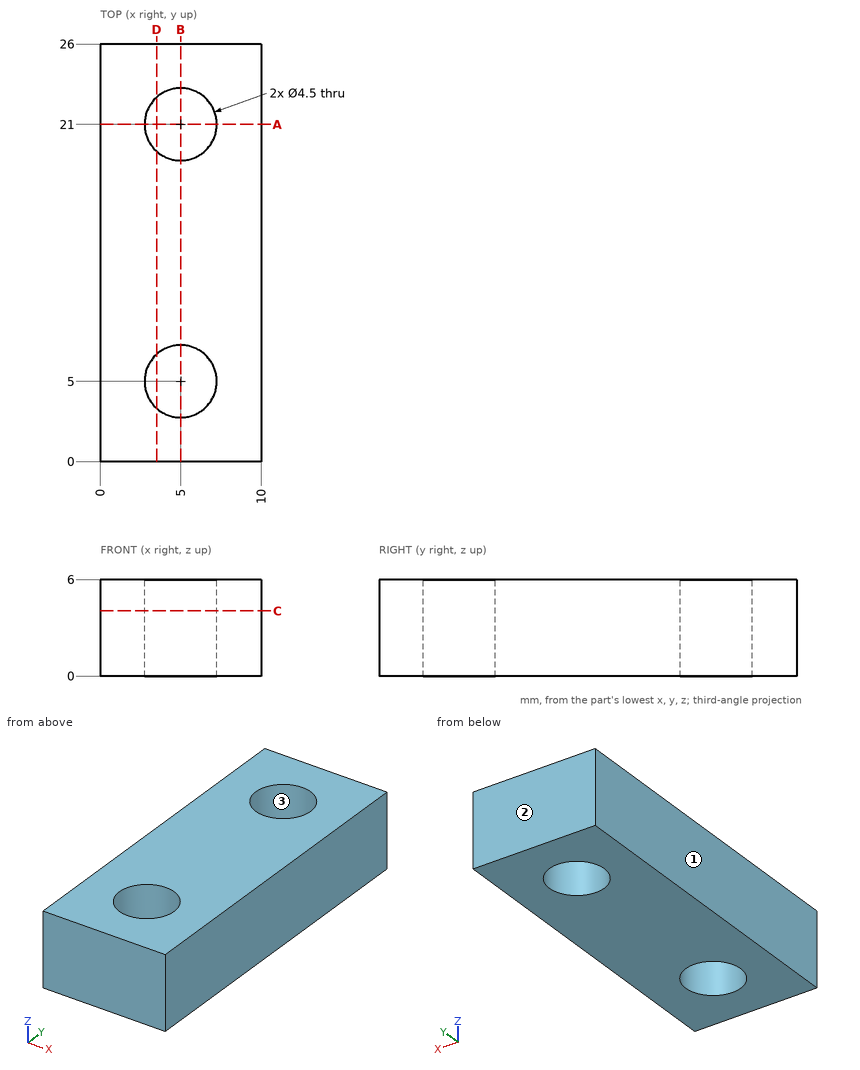
Geometry check sheet. Reference: drawing and pictorial views, mm from the part's lowest x, y, z. Coordinates: 2 decimals unless noted, no trailing zeros. Order: outer loops, then holes, each group sorted by start corner. A loop starts at its lowest first (then second) coordinate and runs counter-clockwise, first axis right, second up.
Item 1: Mould release check, pull along X, two halves, no side actions. Record for the marked faces 1, 2 and 3: released by +X, released by -X, zero draft, split by the parting line, or undercut.
Item 2: Scan lines: line 1 along Y through (x, z) = (5, 2.5); line 2 along Y through (x, z) = (7, 2.85); line 3 along X through (y, z) = (5, 0.65). Record each from-to range of solid material in increasing order.
Item 3: Section check B-B (x = 5). Enter the section's corners in (y, z), plus the area to 3 significant figures.
Item 4: Section check D-D (x = 3.5). Enter the section's corners in (y, z), plus the area to 3 significant figures.
Item 5: Section check A-A (y = 21). Enter the section's corners in (x, z).
Item 6: Section check C-C (z = 4.05). Enter the section's corners in (x, y).
Check sheet entries:
1. face 1: released by -X
1. face 2: zero draft
1. face 3: undercut
2. line 1: y = 0 to 2.75, 7.25 to 18.75, 23.25 to 26
2. line 2: y = 0 to 3.97, 6.03 to 19.97, 22.03 to 26
2. line 3: x = 0 to 2.75, 7.25 to 10
3. outline: (0, 0) - (2.75, 0) - (2.75, 6) - (0, 6) - close; (7.25, 0) - (18.75, 0) - (18.75, 6) - (7.25, 6) - close; (23.25, 0) - (26, 0) - (26, 6) - (23.25, 6) - close
3. area: 102 mm2
4. outline: (0, 0) - (3.32, 0) - (3.32, 6) - (0, 6) - close; (6.68, 0) - (19.32, 0) - (19.32, 6) - (6.68, 6) - close; (22.68, 0) - (26, 0) - (26, 6) - (22.68, 6) - close
4. area: 116 mm2
5. outline: (0, 0) - (2.75, 0) - (2.75, 6) - (0, 6) - close; (7.25, 0) - (10, 0) - (10, 6) - (7.25, 6) - close
6. outline: (0, 0) - (10, 0) - (10, 26) - (0, 26) - close; hole circle Ø4.5 at (5, 5); hole circle Ø4.5 at (5, 21)
